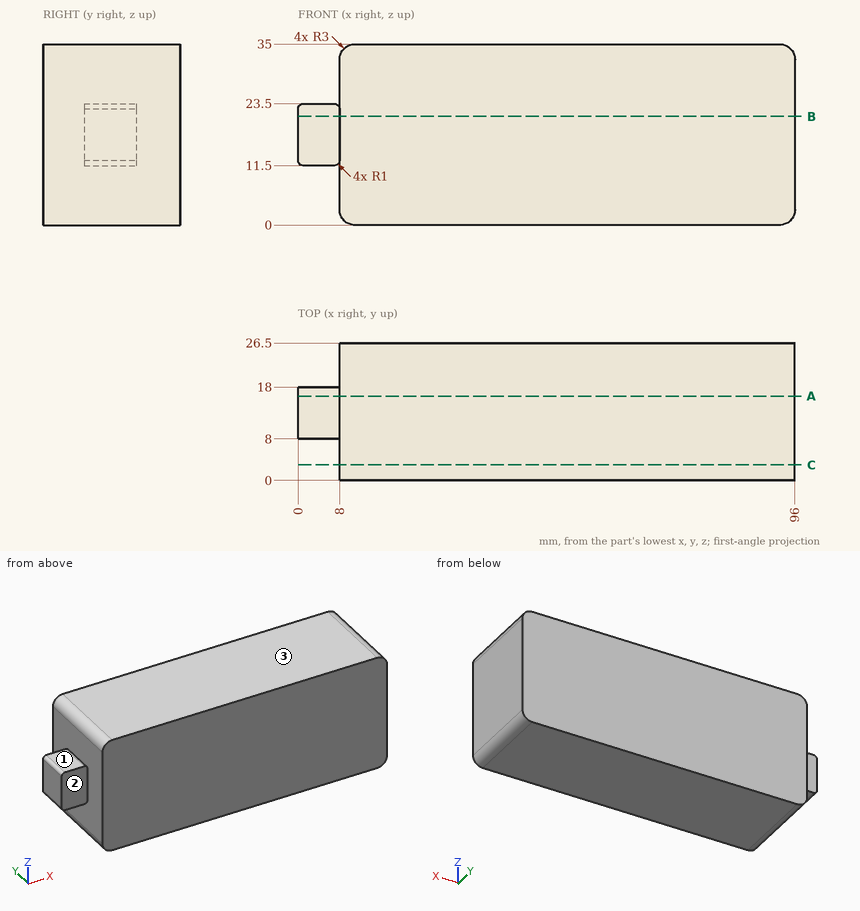
Job drawing, mm, ordinate dimensions from the low corner. One solid piece. A direction names the side the tool comes from. Round coordinates to 2 decimals unless told otherwise and drop trailing zeros. Loops run counter-clockwise (first coordinate to the right, second up) from the corner with the lowest first, then second, coordinate; pieces in that order, holes last.
Item 1: Drop flat-ended pins along their axis: P1, Ø3, axis at y = 7, z = 8, coming from the -X side; P2, Ø2.5, axis at x = 3.5, z = 16.5, coming from the +Y side; P3, Ø6.5, axis at x = 4, y = 11, coming from the +Z side. Give the stop position or say it passes through.
Item 2: Cut at C-C, the plane y = 3. Give the cut face in (x, z), then the cut area to 3 significant figures.
Item 3: Drill centre lines: line 1 (X direction, y = 19.25, z = 27); line 2 (X direction, y = 21.25, z = 34). Where is each one in solid material? Low to high.
Item 4: Cut at A-A, the plane y = 16.25. Give the cut face in (x, z).
Item 5: 3-axis set-ups, long thin cutter, end or side, ignore diameter. For the marked faces 1, 2 and 3: which of +Z, -Z, +X, -X, +Y, -Y reach the whole face in a straight line?
Item 6: Cut at B-B, the plane z = 21. Give the cut face in (x, y), then the cut area to 3 significant figures.
A:
1. P1: stops at x = 8
1. P2: stops at y = 18
1. P3: stops at z = 23.5
2. outline: (8, 3) arc R3 ccw to (11, 0) - (93, 0) arc R3 ccw to (96, 3) - (96, 32) arc R3 ccw to (93, 35) - (11, 35) arc R3 ccw to (8, 32) - close
2. area: 3,070 mm2
3. line 1: x = 8 to 96
3. line 2: x = 8.76 to 95.24
4. outline: (0, 12.5) arc R1 ccw to (1, 11.5) - (7, 11.5) arc R1 ccw to (8, 12.5) - (8, 3) arc R3 ccw to (11, 0) - (93, 0) arc R3 ccw to (96, 3) - (96, 32) arc R3 ccw to (93, 35) - (11, 35) arc R3 ccw to (8, 32) - (8, 22.5) arc R1 ccw to (7, 23.5) - (1, 23.5) arc R1 ccw to (0, 22.5) - close
5. face 1: +Z, -X, +Y, -Y
5. face 2: +Z, -Z, -X, -Y
5. face 3: +Z, +X, -X, +Y, -Y
6. outline: (0, 8) - (8, 8) - (8, 0) - (96, 0) - (96, 26.5) - (8, 26.5) - (8, 18) - (0, 18) - close
6. area: 2,410 mm2
